Build history of the part. All positions in model axes, mm. Give positions to 0.01 mm unless a question says otherwise; leave off trailing zeros. Write each loop counter-clockwise with the first axis right and the second up, starting at its lowest first coordinate (ties: lowest second). Pieces come first, ordered by that corner, then holes. Notation, with made-up numbers: (-36, 58) -> (-27, 58) arc R19 ccw to (-27, 65) -> close; hole circle Ø11 at (-3, 43). An arc over 180 degrees is marked (long way). Write item = value, one per line. Start each with the question number.
Q1. Saw through at A-A, the plane z = 25. List the corners of the cut face in (x, y) (3 decimals), then the cut area to 3 significant figures.
Q2. Saw through at C-C, the plane x = 24.5. List the corners of the cut face in (y, z) (3 decimals), then the cut area to 3 significant figures.
Q3. Wall check: line 1 (Y direction, x = 4.5, z = 117.5) (3 decimals); line 2 (Z direction, x = 35, y = 27). Give the ranges that are in metal, low to high.
from build123d import *

# Parameters (mm, degrees)
SKETCH2_W                = 38.1
SKETCH2_H                = 38.1
SKETCH2_W_2              = 31.75
SKETCH2_H_2              = 31.75
BOSS_EXTRUDE1_DEPTH      = 762
BOSS_EXTRUDE1_DEPTH_BACK = 762
SKETCH3_R                = 21.082
CUT_EXTRUDE1_DEPTH       = 764.902624685
CUT_EXTRUDE2_DEPTH       = 232.775000254


with BuildPart() as part:
    # Sketch2 → Boss-Extrude1 (new, two sides)
    with BuildSketch(Plane.XY) as boss_extrude1_sk:
        with Locations((19.05, 19.05)):
            Rectangle(SKETCH2_W, SKETCH2_H)
        with Locations((19.05, 19.05)):
            Rectangle(SKETCH2_W_2, SKETCH2_H_2, mode=Mode.SUBTRACT)
    extrude(amount=BOSS_EXTRUDE1_DEPTH)
    extrude(boss_extrude1_sk.sketch, amount=-BOSS_EXTRUDE1_DEPTH_BACK)

    # Sketch3 → Cut-Extrude1 (cut, through all)
    with BuildSketch(Plane(origin=(0, 38.1, 0), x_dir=(1, 0, 0), z_dir=(0, 1, 0))):
        with Locations((21.082, -225.425)):
            Circle(SKETCH3_R)
        with Locations((21.082, 225.425)):
            Circle(SKETCH3_R)
    extrude(amount=-CUT_EXTRUDE1_DEPTH, mode=Mode.SUBTRACT)


with BuildPart() as cut_extrude1_kept_piece:
    # of the separate pieces the step leaves, the one the design keeps (cut_extrude1_pieces_kept)
    add(part.part.solids().sort_by_distance((38.1, 38.1, 212.981592107))[0])

    # Sketch4 → Cut-Extrude2 (cut, through all)
    with BuildSketch(Plane(origin=(0, 38.1, 0), x_dir=(1, 0, 0), z_dir=(0, 1, 0))):
        with BuildLine():
            Line((0, -214.3125), (0, -225.425))
            ThreePointArc((0, -225.425), (0.807088464, -219.647570969), (3.166557841, -214.3125))
            Line((3.166557841, -214.3125), (0, -214.3125))
        make_face()
        with BuildLine():
            Line((0, 225.425), (0, 214.3125))
            Line((0, 214.3125), (3.166557841, 214.3125))
            ThreePointArc((3.166557841, 214.3125), (0.807088464, 219.647570969), (0, 225.425))
        make_face()
    extrude(amount=-CUT_EXTRUDE2_DEPTH, mode=Mode.SUBTRACT)


solid = cut_extrude1_kept_piece.part
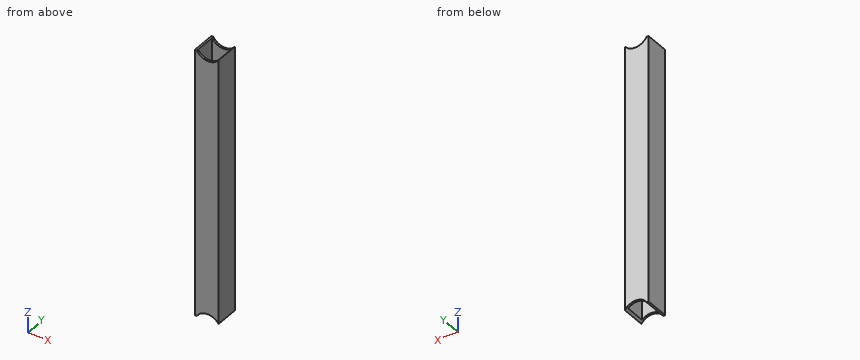
Report:
q1.outline = (0, 0) -> (38.1, 0) -> (38.1, 38.1) -> (0, 38.1) -> close; hole (3.175, 3.175) -> (34.925, 3.175) -> (34.925, 34.925) -> (3.175, 34.925) -> close
q1.area = 444 mm2
q2.outline = (0, -204.622) -> (3.175, -204.622) -> (3.175, 204.622) -> (0, 204.622) -> close; (34.925, -204.622) -> (38.1, -204.622) -> (38.1, 204.622) -> (34.925, 204.622) -> close
q2.area = 2,600 mm2
q3.line_1 = 0 to 3.175, 34.925 to 38.1
q3.line_2 = -209.59 to 209.59
